from build123d import *

# Parameters (mm, degrees)
F1_DEPTH  = 2
F2_W      = 26
F2_H      = 26
F3_DEPTH  = 15.4
F4_W      = 35
F4_H      = 35
F4_W_2    = 37
F5_DEPTH  = 25
F6_W      = 26
F6_H      = 5
F7_DEPTH  = 25
F8_R      = 4
F9_R      = 2
F10_R     = 5
F11_DEPTH = 25
F12_R     = 5
F13_DEPTH = 25
F14_W     = 46
F14_H     = 46
F14_W_2   = 48
F15_DEPTH = 1
F16_R     = 1
F17_R     = 1
F0_W      = 5
F0_H      = 3
F0_W_2    = 3
F0_H_2    = 5
F18_DEPTH = 2


# Not quite as in the source:
# - a feature names something its author has since deleted; it is built from what else it names


with BuildPart() as f1:
    # F0 (on Top) → F1 (new body)
    with BuildSketch(Plane.XY):
        Polygon((172.5389735401, 18.1442317292), (-23.8906879723, 18.1442317292), (-23.8906879723, 13.5384923518), (-23.8906879723, 10.5384923518), (-23.8906879723, -31.8557682708), (-9.5117332786, -31.8557682708), (-6.5117332786, -31.8557682708), (186.1093120277, -31.8557682708), (186.1093120277, -31.4002893865), (186.1093120277, -28.4002893865), (186.1093120277, 18.1442317292), (175.5389735401, 18.1442317292), align=None)
    extrude(amount=F1_DEPTH)

    # F2 (on face) → F3 (cut)
    with BuildSketch(Plane(origin=(0, 0, 0), x_dir=(1, 0, 0), z_dir=(0, 0, -1))):
        with Locations((10.1093120277, 6.8557682708)):
            Rectangle(F2_W, F2_H)
    extrude(amount=-F3_DEPTH, mode=Mode.SUBTRACT)

    # F4 (on face) → F5 (cut)
    with BuildSketch(Plane(origin=(0, 0, 0), x_dir=(1, 0, 0), z_dir=(0, 0, -1))):
        with Locations((67.6093120277, 6.8557682708)):
            Rectangle(F4_W, F4_H)
        with Locations((152.6093120277, 6.8557682708)):
            Rectangle(F4_W_2, F4_H)
    extrude(amount=-F5_DEPTH, mode=Mode.SUBTRACT)

    # F6 (on face) → F7 (cut)
    with BuildSketch(Plane.XY.offset(2)):
        with Locations((10.1093120277, -29.3557682708)):
            Rectangle(F6_W, F6_H)
    extrude(amount=-F7_DEPTH, mode=Mode.SUBTRACT)

    # F8
    f8_edges = [f1.edges().sort_by_distance(p)[0] for p in [
        (-2.890688, -26.855768, 1),
        (23.109312, -26.855768, 1),
    ]]
    fillet(f8_edges, radius=F8_R)

    # F9
    f9_edges = [f1.edges().sort_by_distance(p)[0] for p in [
        (50.109312, 10.644232, 1),
        (85.109312, 10.644232, 1),
        (50.109312, -24.355768, 1),
        (134.109312, -24.355768, 1),
        (85.109312, -24.355768, 1),
        (171.109312, -24.355768, 1),
        (134.109312, 10.644232, 1),
        (171.109312, 10.644232, 1),
        (23.109312, 6.144232, 1),
        (-2.890688, 6.144232, 1),
        (23.109312, -19.855768, 1),
        (-2.890688, -19.855768, 1),
    ]]
    fillet(f9_edges, radius=F9_R)

    # F10 (on face) → F11 (cut)
    with BuildSketch(Plane.XY.offset(2)):
        with Locations((120.1093120277, 11.1442317292)):
            Circle(F10_R)
        with Locations((120.1093120277, -24.8557682708)):
            Circle(F10_R)
        with Locations((31.1093120277, -24.8557682708)):
            Circle(F10_R)
        with Locations((-13.8906879723, 11.1442317292)):
            Circle(F10_R)
        with Locations((-13.8906879723, -24.8557682708)):
            Circle(F10_R)
    extrude(amount=-F11_DEPTH, mode=Mode.SUBTRACT)

    # F12 (on face) → F13 (cut)
    with BuildSketch(Plane.XY.offset(2)):
        with Locations((31.1093120277, 11.1442317292)):
            Circle(F12_R)
    extrude(amount=-F13_DEPTH, mode=Mode.SUBTRACT)

    # F14 (on face) → F15 (cut)
    with BuildSketch(Plane.XY):
        with Locations((67.6093120277, -6.8557682708)):
            Rectangle(F14_W, F14_H)
        with Locations((152.6093120277, -6.8557682708)):
            Rectangle(F14_W_2, F14_H)
    extrude(amount=F15_DEPTH, mode=Mode.SUBTRACT)

    # F16
    f16_edges = [f1.edges().sort_by_distance(p)[0] for p in [
        (44.609312, -29.855768, 0.5),
        (90.609312, -29.855768, 0.5),
        (90.609312, 16.144232, 0.5),
        (44.609312, 16.144232, 0.5),
    ]]
    fillet(f16_edges, radius=F16_R)

    # F17
    f17_edges = [f1.edges().sort_by_distance(p)[0] for p in [
        (128.609312, -29.855768, 0.5),
        (176.609312, -29.855768, 0.5),
        (176.609312, 16.144232, 0.5),
        (128.609312, 16.144232, 0.5),
    ]]
    fillet(f17_edges, radius=F17_R)

    # F0 (on Top) → F18 (join)
    with BuildSketch(Plane.XY):
        with Locations((188.6093120277, -29.9002893865)):
            Rectangle(F0_W, F0_H)
        with Locations((174.0389735401, 20.6442317292)):
            Rectangle(F0_W_2, F0_H_2)
        with Locations((-8.0117332786, -34.3557682708)):
            Rectangle(F0_W_2, F0_H_2)
        with Locations((-26.3906879723, 12.0384923518)):
            Rectangle(F0_W, F0_H)
    extrude(amount=F18_DEPTH)


solid = f1.part
Part model, mm, in its own coordinate system. A direction names the side the tool comes from. Coordinates: 2 decimals unless noted, no trailing zeros. Order: outer loops, then holes, each group sorted by start corner. A loop starts at its lowest first (then second) coordinate and runs counter-clockwise, first axis right, second up. Notation, with made-up numbers: M 82,62 L 133,62 A16 cw 133,74 Z; hole C 81,-36 d6. An arc over 180 degrees is marked long. One line per question, with ' | ' between items.
Q1. Pin check, flat tips, straight feed: P1, Ø0.8, axis at x = 156.5, z = 0.5, coming from the -Y side; P2, Ø16, axis at x = 120.11, y = 11.14, coming from the +Z side; P3, Ø0.5, axis at y = -8.5, z = 0.5, coming from the -X side; P4, Ø1, axis at y = 21, z = 1, coming from the -X side. Stop position of each tip, or through.
A:
P1: stops at y = -31.86 | P2: stops at z = 2 | P3: stops at x = -23.89 | P4: stops at x = 172.54
Q2. 3-axis set-ups, long thin cutter, end or side, ignore diameter. For faces 3 (the face through (152, -27, 1)), 4 (the face through (124.73, 9.23, 1.01)), 5 (the face through (21.97, -28.06, 0.99)): which of +Z, -Z, +X, -X, +Y, -Y reach the whole face in a straight line?
A:
face 3: -Z | face 4: +Z, -Z | face 5: +Z, -Z, -Y
Q3. Slice it at B-B (x = 74). Give the cut face in (y, z), and give its area (3 significant figures).
A:
outline: M -31.86,0 L -29.86,0 L -29.86,1 L -24.36,1 L -24.36,2 L -31.86,2 Z; M 10.64,1 L 16.14,1 L 16.14,0 L 18.14,0 L 18.14,2 L 10.64,2 Z | area: 19.0 mm^2
Q4. Slice it at A-A (y = -11.5). Give the cut face in (x, z), and give its area (3 significant figures).
A:
outline: M -23.89,0 L -2.89,0 L -2.89,2 L -23.89,2 Z; M 23.11,0 L 44.61,0 L 44.61,1 L 50.11,1 L 50.11,2 L 23.11,2 Z; M 85.11,1 L 90.61,1 L 90.61,0 L 128.61,0 L 128.61,1 L 134.11,1 L 134.11,2 L 85.11,2 Z; M 171.11,1 L 176.61,1 L 176.61,0 L 186.11,0 L 186.11,2 L 171.11,2 Z | area: 202 mm^2
Q5. Slice it at C-C (x = 48). Give the cut face in (y, z), and give its area (3 significant figures).
A:
outline: M -31.86,0 L -29.86,0 L -29.86,1 L 16.14,1 L 16.14,0 L 18.14,0 L 18.14,2 L -31.86,2 Z | area: 54.0 mm^2
Q6. Slice it at D-D (x = 121). Give the cut face in (y, z), and give its area (3 significant figures).
A:
outline: M -31.86,0 L -29.78,0 L -29.78,2 L -31.86,2 Z; M -19.94,0 L 6.22,0 L 6.22,2 L -19.94,2 Z; M 16.06,0 L 18.14,0 L 18.14,2 L 16.06,2 Z | area: 60.6 mm^2
Q7. Drill centre lines: line 1 (X direction, y = -2.5, z = 1.55); line 2 (X direction, y = 4, z = 0.3); line 3 (Y direction, x = 76, z = 0.85). Where is each one in solid material? Low to high.
A:
line 1: x = -23.89 to -2.89, 23.11 to 50.11, 85.11 to 134.11, 171.11 to 186.11 | line 2: x = -23.89 to -2.89, 23.11 to 44.61, 90.61 to 128.61, 176.61 to 186.11 | line 3: y = -31.86 to -29.86, 16.14 to 18.14
Q8. Two-plate mould, pull along X, no slides. Class faces 1 (the face through (-1.75, -28.06, 0.99)), 2 (the face through (104, -6, 2)): +X half, -X half, draft (parallel to the pull), parting line (faces both ways), or undercut.
A:
face 1: undercut | face 2: draft
